Autodesk Inventor part; units mm, degrees
ref_plane "YZ Plane" through (0, 0, 0) normal (1, 0, 0) x (0, 1, 0)
ref_plane "XZ Plane" through (0, 0, 0) normal (0, 1, 0) x (-1, 0, 0)
ref_plane "XY Plane" through (0, 0, 0) normal (0, 0, 1) x (1, 0, 0)
sketch "Boceto1" plane through (0, 0, 0) normal (0, 0, 1) x (1, 0, 0)
  line L0 (-70.4693, 87.7725) -> (72.3878, 87.7725) construction
  line L1 (72.3878, 87.7725) -> (72.3878, -52.7037) construction
  line L2 (72.3878, -52.7037) -> (-70.4693, -52.7037) construction
  line L3 (-70.4693, -52.7037) -> (-70.4693, 87.7725) construction
  line L4 (-16, 0) -> (16, 0)
  line L5 (16, 0) -> (16, 4)
  line L6 (16, 4) -> (29, 4)
  line L7 (29, 4) -> (29, 33)
  arc A0 (29, 33) -> (3, 69) centre (-2.439, 37.6829) ccw
  arc A1 (3, 69) -> (-8, 75) centre (-7.5, 62.8333) ccw
  line L8 (-8, 75) -> (-6, 68)
  line L9 (-6, 68) -> (-14, 64)
  line L10 (-14, 64) -> (-16, 58)
  line L11 (-16, 58) -> (-30, 48)
  arc A2 (-30, 48) -> (-23.3333, 36) centre (-21.5351, 44.8509) ccw
  line L12 (-23.3333, 36) -> (-12, 40.4647)
  line L13 (-12, 40.4647) -> (-10, 40)
  line L14 (-10, 40) -> (-2.439, 42.9786)
  arc A3 (-12, 23.8479) -> (-2.439, 42.9786) centre (-19.6735, 39.6374) ccw
  arc A4 (-12, 23.8479) -> (-23.3333, 4) centre (1.7175, 2.8554) ccw
  line L15 (-23.3333, 4) -> (-16, 4)
  line L16 (-16, 4) -> (-16, 0)
  point P0 (0, 0)
extrude "Extrusión1" add sketch "Boceto1" along normal mid plane 10
properties part number "KIGTH TOP 1.0"
Input: part model. Units: mm. Frame: model coordinates. A direction names the side the tool comes from. Round coordinates to 2 decimals unless told otherwise and drop trailing zeros. Loops run counter-clockwise (first coordinate to the right, second up) from the corner with the lowest first, then second, coordinate; pieces in that order, holes last. Notation, with made-up numbers: (-7.5, -32) -> (1.5, -32) arc R16 cw to (1.5, -4) -> close; hole circle Ø10 at (43.25, 72). An arc over 180 degrees is marked (long way). Answer as a JSON object with one key per item and string values. Group by question number.
1) Section query C-C on x = -19.5. Output: boundary loops of the cut face in (y, z).
2) Ray query, L1, parallel to Y at x = -13.5, z = 2.25; L2, parallel to Y at x = 24, z = -4.5; L3, parallel to X at y = 51, z = -1.75. Return the intervals inside material, ascending.
3) Section query A-A on z = 1.5. Output: boundary loops of the cut face in (x, y).
4) Reachability of faces 1 (the flat face through (16, 2, 0)), 2 (the cylindrical face through (-20.14, 15.15, -0.07)), 3 (the flat face through (-20, 4, 0)) from +Z, -Z, +X, -X, +Y, -Y: full face, straight path, thin tool, end or side. Return the list, or none.
5) Section query D-D on x = -25.5. Output: boundary loops of the cut face in (y, z).
6) Pin query (flat end, axial travel): pin 1 (3 mm diameter, centred on y = 1.5, z = -2, fed in from +X); pin 2 (1.2 mm diameter, centred on y = 3, z = 0.5, fed in from -X); pin 3 (2 mm diameter, centred on y = 34, z = 0, fed in from -X). Return the tip coordinate at first contact, or that it passes through.
7) Draft query along X for faces 4 (the flat face through (6, 30, -5)), 5 (the flat face through (-17.75, 38.2, -0.07)), 6 (the cylindrical face through (-29.377, 40.37, -0.07)). Return one class per face: +X half, -X half, draft (parallel to the pull), parting line (faces both ways), or undercut.
8) Section query B-B on y = 38.5. Output: boundary loops of the cut face in (x, z) (3 decimals).
Reply:
{
 "1": {"outline": "(4, -5) -> (16.22, -5) -> (16.22, 5) -> (4, 5) -> close; (37.51, -5) -> (55.5, -5) -> (55.5, 5) -> (37.51, 5) -> close"},
 "2": {"L1": "y = 0 to 22.79, 39.87 to 64.25", "L2": "y = 4 to 55.33", "L3": "x = -25.8 to 26.42"},
 "3": {"outline": "(-30, 48) arc R9.03 ccw to (-23.33, 36) -> (-12, 40.46) -> (-10, 40) -> (-2.44, 42.98) arc R17.56 cw to (-12, 23.85) arc R25.08 ccw to (-23.33, 4) -> (-16, 4) -> (-16, 0) -> (16, 0) -> (16, 4) -> (29, 4) -> (29, 33) arc R31.79 ccw to (3, 69) arc R12.18 ccw to (-8, 75) -> (-6, 68) -> (-14, 64) -> (-16, 58) -> close"},
 "4": {"face 1": "+Z, -Z, +X, -Y", "face 2": "+Z, -Z, -X", "face 3": "+Z, -Z, -X, -Y"},
 "5": {"outline": "(36.74, -5) -> (51.21, -5) -> (51.21, 5) -> (36.74, 5) -> close"},
 "6": {"pin 1": "stops at x = 16", "pin 2": "stops at x = -16", "pin 3": "stops at x = -3.42"},
 "7": {"face 4": "draft", "face 5": "undercut", "face 6": "-X half"},
 "8": {"outline": "(-27.957, -5) -> (-16.987, -5) -> (-16.987, 5) -> (-27.957, 5) -> close; (-2.155, -5) -> (29.336, -5) -> (29.336, 5) -> (-2.155, 5) -> close"}
}
